Source: CAD feature listing. Evaluate the final solid. Frame: model axes, mm. A direction names the side the tool comes from. Give positions to 0.01 mm unless a question says otherwise; leave off trailing zeros. Order: outer loops, then holes, each group sorted by start corner. A loop starts at its lowest first (then second) coordinate and runs counter-clockwise, first axis right, second up. Notation, with made-up numbers: M -24.5,53 L 8.5,53 A22 ccw 8.5,86 Z; hole C 30,11 d1. An arc over 180 degrees is marked long. Answer as a JSON object with one key per item and string values. Group by question number.
1. Material intervals for L1, parallel to X at y = 1.25, z = 1.25; L2, parallel to Z at x = 0.65, y = 0.45; L3, parallel to X at y = -0.1, z = 2, sorted ascending. Write a range as [from, to].
2. Pin query (flat end, axial travel): P1, Ø1, axis at x = 0, y = 1, coming from the -Z side; P2, Ø1, axis at x = -1, z = 0.5, coming from the -Y side. Return the tip coordinate at first contact, or that it passes through.
3. Set-up query: faces 1 (the cylindrical face through (-0.75, 0.03, 3.17)), 2 (the cylindrical face through (-0.75, 0.03, -1.61)). Return all of +Z, -Z, +X, -X, +Y, -Y with unobstructed straight access to the full face (end or side cutting, diameter ignored); none if empty.
4. Section query A-A (z = -1.5). Output: boundary loops of the cut face in (x, y), plus the area to 3 significant figures.
from build123d import *

# Parameters (mm, degrees)
SKETCH1_R                = 0.75
BOSS_EXTRUDE1_DEPTH      = 2.4
BOSS_EXTRUDE2_DEPTH      = 4.7124
BOSS_EXTRUDE2_DEPTH_BACK = 3.927
SKETCH1_2_R              = 0.75
CHAMFER1_SIZE            = 0.75


with BuildPart() as part:
    # Sketch1 → Boss-Extrude1 (new body)
    with BuildSketch(Plane.XY):
        with BuildLine():
            Line((-0.103544507, 0.982056406), (-0.131068996, 1.243109375))
            ThreePointArc((-0.131068996, 1.243109375), (-0.10199222, 1.373586424), (0, 1.46))
            ThreePointArc((0, 1.46), (0.10199222, 1.373586424), (0.131068996, 1.243109375))
            Line((0.131068996, 1.243109375), (0.103544507, 0.982056406))
            ThreePointArc((0.103544507, 0.982056406), (0.305154282, 0.93916831), (0.493469007, 0.855362256))
            Line((0.493469007, 0.855362256), (0.624644312, 1.082737033))
            ThreePointArc((0.624644312, 1.082737033), (0.724860403, 1.171204283), (0.858166468, 1.181164812))
            ThreePointArc((0.858166468, 1.181164812), (0.889887282, 1.051305237), (0.836718403, 0.928656187))
            Line((0.836718403, 0.928656187), (0.661007538, 0.733638388))
            ThreePointArc((0.661007538, 0.733638388), (0.798904282, 0.580437937), (0.901994132, 0.401948797))
            Line((0.901994132, 0.401948797), (1.141764724, 0.508795946))
            ThreePointArc((1.141764724, 0.508795946), (1.27484099, 0.521461914), (1.388542514, 0.451164812))
            ThreePointArc((1.388542514, 0.451164812), (1.337875649, 0.327461182), (1.222769819, 0.2594879))
            Line((1.222769819, 0.2594879), (0.965988157, 0.204995441))
            ThreePointArc((0.965988157, 0.204995441), (0.9875, 0), (0.965988157, -0.204995441))
            Line((0.965988157, -0.204995441), (1.222769819, -0.2594879))
            ThreePointArc((1.222769819, -0.2594879), (1.337875649, -0.327461182), (1.388542514, -0.451164812))
            ThreePointArc((1.388542514, -0.451164812), (1.27484099, -0.521461914), (1.141764724, -0.508795946))
            Line((1.141764724, -0.508795946), (0.901994132, -0.401948797))
            ThreePointArc((0.901994132, -0.401948797), (0.798904282, -0.580437937), (0.661007538, -0.733638388))
            Line((0.661007538, -0.733638388), (0.836718403, -0.928656187))
            ThreePointArc((0.836718403, -0.928656187), (0.889887282, -1.051305237), (0.858166468, -1.181164812))
            ThreePointArc((0.858166468, -1.181164812), (0.724860403, -1.171204283), (0.624644312, -1.082737033))
            Line((0.624644312, -1.082737033), (0.493469007, -0.855362256))
            ThreePointArc((0.493469007, -0.855362256), (0.305154282, -0.93916831), (0.103544507, -0.982056406))
            Line((0.103544507, -0.982056406), (0.131068996, -1.243109375))
            ThreePointArc((0.131068996, -1.243109375), (0.10199222, -1.373586424), (0, -1.46))
            ThreePointArc((0, -1.46), (-0.10199222, -1.373586424), (-0.131068996, -1.243109375))
            Line((-0.131068996, -1.243109375), (-0.103544507, -0.982056406))
            ThreePointArc((-0.103544507, -0.982056406), (-0.305154282, -0.93916831), (-0.493469007, -0.855362256))
            Line((-0.493469007, -0.855362256), (-0.624644312, -1.082737033))
            ThreePointArc((-0.624644312, -1.082737033), (-0.724860403, -1.171204283), (-0.858166468, -1.181164812))
            ThreePointArc((-0.858166468, -1.181164812), (-0.889887282, -1.051305237), (-0.836718403, -0.928656187))
            Line((-0.836718403, -0.928656187), (-0.661007538, -0.733638388))
            ThreePointArc((-0.661007538, -0.733638388), (-0.798904282, -0.580437937), (-0.901994132, -0.401948797))
            Line((-0.901994132, -0.401948797), (-1.141764724, -0.508795946))
            ThreePointArc((-1.141764724, -0.508795946), (-1.27484099, -0.521461914), (-1.388542514, -0.451164812))
            ThreePointArc((-1.388542514, -0.451164812), (-1.337875649, -0.327461182), (-1.222769819, -0.2594879))
            Line((-1.222769819, -0.2594879), (-0.965988157, -0.204995441))
            ThreePointArc((-0.965988157, -0.204995441), (-0.9875, 0), (-0.965988157, 0.204995441))
            Line((-0.965988157, 0.204995441), (-1.222769819, 0.2594879))
            ThreePointArc((-1.222769819, 0.2594879), (-1.337875649, 0.327461182), (-1.388542514, 0.451164812))
            ThreePointArc((-1.388542514, 0.451164812), (-1.27484099, 0.521461914), (-1.141764724, 0.508795946))
            Line((-1.141764724, 0.508795946), (-0.901994132, 0.401948797))
            ThreePointArc((-0.901994132, 0.401948797), (-0.798904282, 0.580437937), (-0.661007538, 0.733638388))
            Line((-0.661007538, 0.733638388), (-0.836718403, 0.928656187))
            ThreePointArc((-0.836718403, 0.928656187), (-0.889887282, 1.051305237), (-0.858166468, 1.181164812))
            ThreePointArc((-0.858166468, 1.181164812), (-0.724860403, 1.171204283), (-0.624644312, 1.082737033))
            Line((-0.624644312, 1.082737033), (-0.493469007, 0.855362256))
            ThreePointArc((-0.493469007, 0.855362256), (-0.305154282, 0.93916831), (-0.103544507, 0.982056406))
        make_face()
        Circle(SKETCH1_R, mode=Mode.SUBTRACT)
    extrude(amount=BOSS_EXTRUDE1_DEPTH)

    # Sketch1<2> → Boss-Extrude2 (add, two sides: drawn at the far end of the back side and taken through both)
    with BuildSketch(Plane.XY.offset(-BOSS_EXTRUDE2_DEPTH_BACK)):
        Circle(SKETCH1_2_R)
    extrude(amount=BOSS_EXTRUDE2_DEPTH + BOSS_EXTRUDE2_DEPTH_BACK)

    # Chamfer1
    chamfer1_edges = [part.edges().sort_by_distance(p)[0] for p in [
        (-0.75, 0, -3.927),
        (-0.75, 0, 4.7124),
    ]]
    chamfer(chamfer1_edges, length=CHAMFER1_SIZE)


solid = part.part
Answer sheet:
{
 "1": {"L1": "[-0.13, 0.13]", "L2": "[0, 2.4]", "L3": "[-0.98, 0.98]"},
 "2": {"P1": "z = -3.43", "P2": "y = -1.19"},
 "3": {"face 1": "+Z", "face 2": "-Z"},
 "4": {"outline": "C 0,0 d1.5", "area": "1.77 mm^2"}
}
